The listing builds one solid part. Answer for the finished solid, in the listing's coordinates (mm). Face numbers are marked on the shaded views. A direction names the side the tool comes from. Round coordinates to 2 decimals unless told otherwise and drop trailing zeros. Order: outer loops, then holes, each group sorted by start corner. A loop starts at its lowest first (then second) coordinate and runs counter-clockwise, first axis right, second up. Notation, with made-up numbers: (1.5, 73.5) -> (46.5, 73.5) arc R4 cw to (46.5, 79.5) -> close; hole circle Ø2 at (55, -23.75). An arc over 180 degrees is marked (long way). Return JSON: item names as keys, results as strings. Group by question number.
(1) Determine the mould class of the marked faces 3, 4 and 5 for opening direction Z: +Z half, -Z half, draft (parallel to the pull), parting line (faces both ways), or undercut.
(2) Each of these flat-tipped pins is pushed along its axis until it touches: pin 1 (2 mm diameter, centred on x = 3, z = 9, fed in from -Y); pin 2 (3 mm diameter, centred on x = 5.5, z = 4.5, fed in from +Y); pin 3 (8 mm diameter, centred on x = -1, z = -1.5, fed in from +Y). Where does it stop, or does it pass through?
(3) Consider line 1 (Y direction, x = -1, z = 5.5); line 2 (Y direction, x = 5.5, z = 3.25); line 3 (Y direction, x = -8.25, z = 7.25). Determine where each line is inside the solid, lowest interval first. Write a range as [from, to].
(4) The part is cut by section A-A (x = 0). Determine the outline of the cut face in (y, z), plus the area to 3 significant figures.
(5) Which of the six approach directions +Z, -Z, +X, -X, +Y, -Y give full straight-line access (tool end or side, diameter ignored) to the marked faces 1 and 2?
(6) The part is cut by section B-B (y = 2.5). Determine the outline of the cut face in (x, z), plus the area to 3 significant figures.
from build123d import *

# Parameters (mm, degrees)
BOSS_EXTRU_1_DEPTH  = 1
SKETCH1_R           = 6.75
BOSS_EXTRUDE1_DEPTH = 20


with BuildPart() as part:
    # Esquisse1 → Révolution1 (revolve)
    with BuildSketch(Plane.XY):
        with BuildLine():
            Line((0, 0), (5, 0))
            Line((5, 0), (14.396926208, 3.420201433))
            ThreePointArc((14.396926208, 3.420201433), (14.728803197, 3.934870166), (14.322587886, 4.393144497))
            Line((14.322587886, 4.393144497), (5, 1))
            Line((5, 1), (0, 1))
            Line((0, 1), (0, 0))
        make_face()
    revolve(axis=Axis((0, 0, 0), (0, 1, 0)))

    # Esquisse2 → Boss.-Extru.1 (add)
    with BuildSketch(Plane.XZ):
        Polygon((2.792425312, -4.14757289), (4.988116143, 0.344524813), (2.195690831, 4.492097703), (-2.792425312, 4.14757289), (-4.988116143, -0.344524813), (-2.195690831, -4.492097703), align=None)
    extrude(amount=BOSS_EXTRU_1_DEPTH)

    # Sketch1 → Boss-Extrude1 (add)
    with BuildSketch(Plane.XZ.offset(1)):
        Circle(SKETCH1_R)
    extrude(amount=BOSS_EXTRUDE1_DEPTH)


solid = part.part
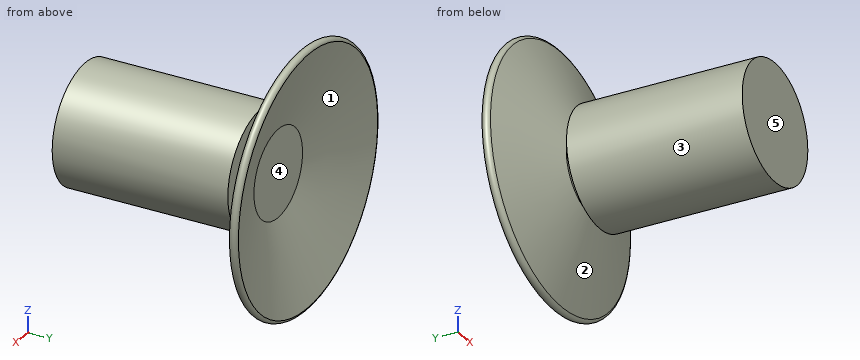
Answer below:
{
 "1": {"face 3": "parting line", "face 4": "undercut", "face 5": "draft"},
 "2": {"pin 1": "stops at y = 1.27", "pin 2": "stops at y = 2.31", "pin 3": "stops at y = 1.29"},
 "3": {"line 1": "y = [-21, -1], [0.21, 1.21]", "line 2": "y = [-21, -1], [0.51, 1.51]", "line 3": "y = [2.18, 3.18]"},
 "4": {"outline": "(-21, -6.75) -> (-1, -6.75) -> (-1, -4.34) -> (0, -4.34) -> (0, -5) -> (3.42, -14.4) arc R0.51 ccw to (4.39, -14.32) -> (1, -5) -> (1, 5) -> (4.39, 14.32) arc R0.51 ccw to (3.42, 14.4) -> (0, 5) -> (0, 4.34) -> (-1, 4.34) -> (-1, 6.75) -> (-21, 6.75) -> close", "area": "308 mm²"},
 "5": {"face 1": "+Y", "face 2": "none"},
 "6": {"outline": "circle Ø23.74 at (0, 0); hole circle Ø18.24 at (0, 0)", "area": "181 mm²"}
}
